Autodesk Inventor part; units mm, degrees
ref_plane "YZ Plane" through (0, 0, 0) normal (1, 0, 0) x (0, 1, 0)
ref_plane "XZ Plane" through (0, 0, 0) normal (0, 1, 0) x (-1, 0, 0)
ref_plane "XY Plane" through (0, 0, 0) normal (0, 0, 1) x (1, 0, 0)
sketch "スケッチ1" plane through (0, 0, 0) normal (0, 1, 0) x (-1, 0, 0)
  circle A0 centre (0, 0) radius 3.5
  circle A1 centre (0, 14.5) radius 2
  circle A2 centre (0, -14.5) radius 2
  line L0 (2, 14.5) -> (2, 2.8723)
  line L1 (-2, 14.5) -> (-2, 2.8723)
  line L2 (-2, -2.8723) -> (-2, -14.5)
  line L3 (2, -2.8723) -> (2, -14.5)
  dimension "d0" = 7
  dimension "d2" = 4
  dimension "d3" = 14.5
  dimension "d4" = 14.5
extrude "押し出し1" add sketch "スケッチ1" along normal blind 1
sketch "スケッチ2" plane through (0, 1, 0) normal (0, 1, 0) x (1, 0, 0)
  arc A0 (-2, 2.8723) -> (-2, -2.8723) centre (0, 0) ccw
  circle A1 centre (0, 0) radius 3.5
extrude "押し出し2" add sketch "スケッチ2" along normal blind 3.5
sketch "スケッチ3" plane through (0, 0, 0) normal (0, -1, 0) x (1, 0, 0)
  arc A0 (2, 14.5) -> (-2, 14.5) centre (0, 14.5) ccw
  point P0 (0, 12.5)
  point P1 (0, 10.5)
  point P2 (0, 8.5)
  point P3 (0, 6.5)
  point P4 (0, 4.5)
  dimension "d9" = 2
  dimension "d18" = 2
  dimension "d19" = 2
  dimension "d20" = 2
  dimension "d21" = 2
hole "穴1" at (0, 0, 14.5) at (0, 0, 12.5) at (0, 0, 10.5) at (0, 0, 8.5) at (0, 0, 6.5) at (0, 0, 4.5) direction (0, 1, 0) diameter 1 end through all
mirror "ミラー1" about plane through (0, 0, 0) normal (0, 0, 1) of "穴1"
properties part number "horn_10g"
The listing builds one solid part. Answer for the finished solid, in the listing's coordinates (mm). A direction names the side the tool comes from. Give positions to 0.01 mm unless a question says otherwise; leave off trailing zeros. Loops run counter-clockwise (first coordinate to the right, second up) from the corner with the lowest first, then second, coordinate; pieces in that order, holes last.
Item 1: A cutting plane is placed at A-A (z = -6.5). Give the vertices of the cut face in (x, y).
Derived:
outline: (-2, 0) - (-0.5, 0) - (-0.5, 1) - (-2, 1) - close; (0.5, 0) - (2, 0) - (2, 1) - (0.5, 1) - close
Item 2: A cutting plane is placed at B-B (y = 0.7). Give the number of separate pieces and of enclosed holes in the cut face, then the cut area to 3 significant figures.
Derived:
separate pieces: 1
enclosed holes: 12
area: 131 mm2
Item 3: A cutting plane is placed at D-D (z = -1). Give the vertices of the cut face in (x, y), then the cut area to 3 significant figures.
Derived:
outline: (-3.35, 0) - (3.35, 0) - (3.35, 4.5) - (-3.35, 4.5) - close
area: 30.2 mm2
Item 4: A cutting plane is placed at C-C (x = -2.5). Give the vertices of the cut face in (y, z).
Derived:
outline: (0, -2.45) - (4.5, -2.45) - (4.5, 2.45) - (0, 2.45) - close
Item 5: Each of these flat-tipped pins is pushed along its axis until it touches: pin 1 Ø3 at (x, z) = (1, 11) entering from +Y; pin 2 Ø0.8 at (y, z) = (0.5, -6) entering from -X; pin 3 Ø0.8 at (y, z) = (0.5, 8) entering from +X. Where does it stop, or does it pass through?
Derived:
pin 1: stops at y = 1
pin 2: stops at x = -2
pin 3: stops at x = 2
Item 6: Find the intervals of material crossed by line 1 along X through (y, z) = (0.35, 10.5); line 2 along Y through (x, z) = (-1.25, 7); line 3 along Z through (x, y) = (0, 2.2), in increasing order.
Derived:
line 1: x = -2 to -0.5, 0.5 to 2
line 2: y = 0 to 1
line 3: z = -3.5 to 3.5
Item 7: A tool of negligible diameter and unlimited length cuts with its end or side. For faces 5 (the cylindrical face through (0.192, 0.507, 8.038)), 6 (the flat face through (-2, 0.5, 8.8)), from which of +Z, -Z, +X, -X, +Y, -Y can it reach the whole face along a straight path? Write none if from no direction.
Derived:
face 5: +Y, -Y
face 6: +Z, -X, +Y, -Y
Item 8: Determine the mould class of faces 1 (the flat face through (2, 0.5, -8.6)), 2 (the cylindrical face through (0, 0.5, 13)), 3 (the cylindrical face through (3.5, 2.2, -0.1)), 4 (the cylindrical face through (-3.5, 2.7, 0)) for opening direction X: +X half, -X half, draft (parallel to the pull), parting line (faces both ways), or undercut.
Derived:
face 1: +X half
face 2: undercut
face 3: parting line
face 4: -X half
